```python
from build123d import *

# Parameters (mm, degrees)
EXTRUDE_1_DEPTH     = 9.5
SKETCH_2_R          = 3
CUT_EXTRUDE_1_DEPTH = 40.542790152
EXTRUDE_START       = 3.5
SKETCH_3_R          = 6
EXTRUDE_2_DEPTH     = 3.5
SKETCH_4_R          = 2.5
CUT_EXTRUDE_2_DEPTH = 41.526315562
SKETCH_5_R          = 5
CUT_EXTRUDE_3_DEPTH = 5
SKETCH_6_R          = 2
CUT_EXTRUDE_4_DEPTH = 40.542790152
SKETCH_8_R          = 4
CUT_EXTRUDE_5_DEPTH = 6
FILLET_1_R          = 6


with BuildPart() as part:
    # 草图1 → 凸台-拉伸1 (new body)
    with BuildSketch(Plane.XY):
        with BuildLine():
            Line((-10, 0), (-10, 9.320888862))
            Line((-10, 9.320888862), (-12.855752194, 9.320888862))
            ThreePointArc((-12.855752194, 9.320888862), (-18.853850562, 15.169839333), (-13.157755506, 21.313283542))
            Line((-13.157755506, 21.313283542), (24.272558016, 23.19968777))
            ThreePointArc((24.272558016, 23.19968777), (30.572659697, 17.35834262), (24.574561329, 11.207293091))
            Line((24.574561329, 11.207293091), (10, 11.207293091))
            Line((10, 11.207293091), (10, 0))
            ThreePointArc((10, 0), (0, -10), (-10, 0))
        make_face()
    extrude(amount=EXTRUDE_1_DEPTH)

    # 草图2 → 切除-拉伸1 (cut, through all)
    with BuildSketch(Plane(origin=(0, 0, 0), x_dir=(-1, 0, 0), z_dir=(0, 0, -1))):
        Circle(SKETCH_2_R)
    extrude(amount=-CUT_EXTRUDE_1_DEPTH, mode=Mode.SUBTRACT)

    # 草图3 → 凸台-拉伸2 (add)
    with BuildSketch(Plane(origin=(0, 0, 0), x_dir=(-1, 0, 0), z_dir=(0, 0, -1)).offset(EXTRUDE_START)):
        with Locations((-24.574561329, 17.207293091)):
            Circle(SKETCH_3_R)
    extrude(amount=-EXTRUDE_2_DEPTH)

    # 草图4 → 切除-拉伸2 (cut, through all)
    with BuildSketch(Plane(origin=(0, 0, -3.5), x_dir=(-1, 0, 0), z_dir=(0, 0, -1))):
        with Locations((-24.574561329, 17.207293091)):
            Circle(SKETCH_4_R)
    extrude(amount=-CUT_EXTRUDE_2_DEPTH, mode=Mode.SUBTRACT)

    # 草图5 → 切除-拉伸3 (cut)
    with BuildSketch(Plane.XY.offset(9.5)):
        with Locations((24.574561329, 17.207293091)):
            Circle(SKETCH_5_R)
    extrude(amount=-CUT_EXTRUDE_3_DEPTH, mode=Mode.SUBTRACT)

    # 草图6 → 切除-拉伸4 (cut, through all)
    with BuildSketch(Plane(origin=(0, 0, 0), x_dir=(-1, 0, 0), z_dir=(0, 0, -1))):
        with Locations((12.855752194, 15.320888862)):
            Circle(SKETCH_6_R)
    extrude(amount=-CUT_EXTRUDE_4_DEPTH, mode=Mode.SUBTRACT)

    # 草图8 → 切除-拉伸5 (cut)
    with BuildSketch(Plane(origin=(0, 0, 0), x_dir=(-1, 0, 0), z_dir=(0, 0, -1))):
        with Locations((12.855752194, 15.320888862)):
            Circle(SKETCH_8_R)
    extrude(amount=-CUT_EXTRUDE_5_DEPTH, mode=Mode.SUBTRACT)

    # 圆角1
    fillet_1_edges = [part.edges().sort_by_distance(p)[0] for p in [
        (-10, 9.320888862, 4.75),
        (10, 11.207293091, 4.75),
    ]]
    fillet(fillet_1_edges, radius=FILLET_1_R)


solid = part.part
```
Read the model definition and answer for the solid it produces. Units are mm, in the model's axes. A direction names the side the tool comes from. Give positions to 0.01 mm unless a question says otherwise; leave off trailing zeros. Order: outer loops, then holes, each group sorted by start corner. A loop starts at its lowest first (then second) coordinate and runs counter-clockwise, first axis right, second up.
(1) Straight lines are drawn through the part: L1, parallel to X at y = 15.5, z = 1.25; L2, parallel to X at y = 15.5, z = 8.25; L3, parallel to Z at x = -7.5, y = 12.5. For each, find the intervals that lie inside material, in ascending order.
(2) Find section C-C (z = 6.5). Give the number of separate pieces and of enclosed holes in the cut face, plus the area to 3 significant figures.
(3) Given pin 1 (1.5 mm diameter, centred on x = -3, z = -0.5, fed in from +Y); pin 2 (6.5 mm diameter, centred on x = 24.57, y = 17.21, fed in from +Z); pin 3 (4 mm diameter, centred on y = 2.5, z = 3, fed in from -X), each flat-ended and moving along its own axis, determine where each tip first touches the part or whether it passes through.
(4) For faces 1 (the cylindrical face through (29.344, 18.709, 7.035)), 2 (the flat face through (20, 11.207, 5)), 3 (the flat face through (-11, 14, 6)), determine the directions among +Z, -Z, +X, -X, +Y, -Y from which every point of the face is accessible in a straight line to the end or side of a thin tool.
(5) For a pull along Y with two mould halves and no side action, classify faces 4 (the flat face through (22, 16, 4.5)), 5 (the flat face through (-10, 2, 5)), 6 (the flat face through (5.295, 22.243, 4.684)), 7 (the cylindrical face through (0, -10, 5)) as released by +Y, released by -Y, zero draft, split by the parting line, or undercut.
(6) Find section D-D (x = 14). Give the vertices of the cut face in (y, z), plus the area to 3 significant figures.
(7) Find section A-A (x = 0). Give the vertices of the cut face in (y, z).
(8) Find section B-B (y = -2). Give the vertices of the cut face in (x, z), plus the area to 3 significant figures.
Result sheet:
1. L1: x = -18.85 to -16.85, -8.86 to 22.75, 26.4 to 30.33
1. L2: x = -18.85 to -14.85, -10.86 to 19.88, 29.27 to 30.33
1. L3: z = 0 to 9.5
2. separate pieces: 1
2. enclosed holes: 3
2. area: 808 mm2
3. pin 1: stops at y = 21.85
3. pin 2: stops at z = 4.5
3. pin 3: stops at x = -10.05
4. face 1: +Z
4. face 2: +Z, -Z, +X, -Y
4. face 3: -Z
5. face 4: undercut
5. face 5: zero draft
5. face 6: released by +Y
5. face 7: released by -Y
6. outline: (10.86, 0) - (22.68, 0) - (22.68, 9.5) - (10.86, 9.5) - close
6. area: 112 mm2
7. outline: (-10, 0) - (-3, 0) - (-3, 9.5) - (-10, 9.5) - close; (3, 0) - (21.98, 0) - (21.98, 9.5) - (3, 9.5) - close
8. outline: (-9.8, 0) - (-2.24, 0) - (-2.24, 9.5) - (-9.8, 9.5) - close; (2.24, 0) - (9.8, 0) - (9.8, 9.5) - (2.24, 9.5) - close
8. area: 144 mm2
